Design review of the part shown in the three views and the two pictorial views. Dimensions are in mm from the part's minimum x, y and z. A direction names the side the tool comes from. Give positions to 0.01 mm unless a question says otherwise; leave off trailing zeros. Loops run counter-clockwise (first coordinate to the right, second up) from the corner with the lowest first, then second, coordinate; pieces in that order, holes last.
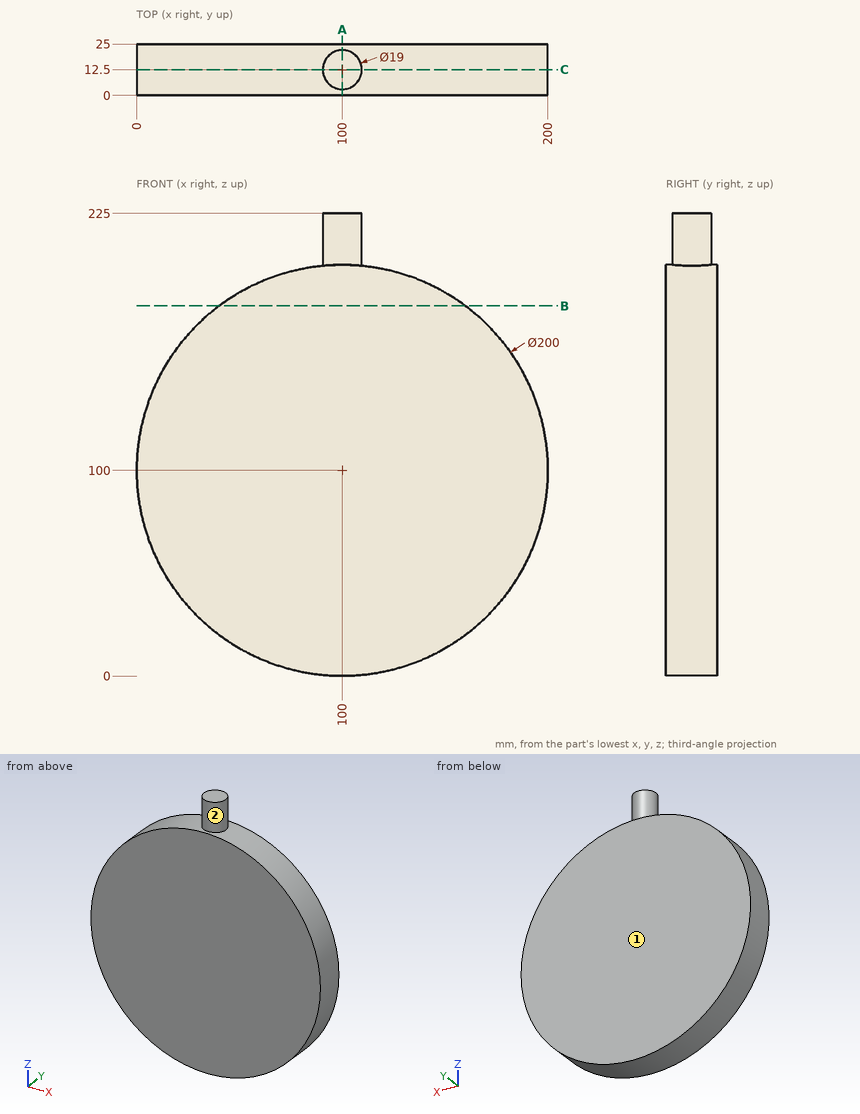
Q1. Wall thickness on line 1 (X direction, y = 14, z = 91); line 2 (Z direction, x = 64.5, y = 6.25); line 3 (X direction, y = 22.25, z = 92): over which ranges is each line inside the solid? List them lowest first.
Results:
line 1: x = 0.41 to 199.59
line 2: z = 6.51 to 193.49
line 3: x = 0.32 to 199.68
Q2. Tool access review of the marked faces 1 and 2: name each direction out of +Z, -Z, +X, -X, +Y, -Y from which nothing blocks a thin tool from reaching the whole face with its end or side.
Results:
face 1: +Z, -Z, +X, -X, +Y
face 2: +Z
Q3. Take a section at C-C (y = 12.5). Give the boundary of the cut face in (x, z), plus the area to 3 significant figures.
Results:
outline: (90.5, 199.55) arc R100 ccw (long way) to (109.5, 199.55) - (109.5, 225) - (90.5, 225) - close
area: 31,900 mm2
Q4. Take a section at A-A (x = 100). Give the boundary of the cut face in (y, z), plus the area to 4 significant figures.
Results:
outline: (0, 0) - (25, 0) - (25, 200) - (22, 200) - (22, 225) - (3, 225) - (3, 200) - (0, 200) - close
area: 5,475 mm2
Q5. Take a section at B-B (z = 180). Give the boundary of the cut face in (x, y).
Results:
outline: (40, 0) - (160, 0) - (160, 25) - (40, 25) - close
Q6. Insertion check: pin 1 (5 mm diameter, centred on x = 76, y = 9, fed in from +Z); pin 2 (6 mm diameter, centred on x = 37, y = 22, fed in from -Z); pin 3 (8 mm diameter, centred on x = 139, y = 17, fed in from +Z) (3 decimals). Each pin has a flat end and moves straight along its axis. Give the tip position at first contact, or say it passes through.
Results:
pin 1: stops at z = 197.66
pin 2: stops at z = 20
pin 3: stops at z = 193.675
